Study the drawing (mm; zero at the part's minimum x, y, z) and answer. Coordinates: 2 decimals unless noted, no trailing zeros. Loops run counter-clockwise (first coordinate to the right, second up) from the corner with the lowest first, then second, coordinate; pieces in that order, holes last. Notation, with made-up numbers: (38, 50) - (97, 50) arc R13 ccw to (97, 69) - close; hole circle Ø5 at (-35.75, 67). An arc over 180 degrees is marked (long way). Write each question's results on one line, items separated by ' | '. Start each with the question number.
(1) Find section B-B on x = 59. Determine the outline of the cut face in (y, z).
(2) Given pin 1 Ø2 at (x, z) = (91, 48) entering from -Y; pin 2 Ø1.5 at (x, z) = (64, 31.5) entering from -Y, each flat-ended and moving along its own axis, determine where each tip first touches the part or whether it passes through.
(3) Find section D-D on x = 5. Determine the outline of the cut face in (y, z), then the cut area to 3 significant figures.
(4) Find section C-C on y = 1.8. State how many separate pieces and enclosed holes the cut face has, then the cut area to 3 significant figures.
(5) Consider line 1 (X direction, y = 3.3, z = 48); line 2 (Z direction, x = 81, y = 2.7); line 3 (X direction, y = 1.85, z = 26). Determine where each line is inside the solid, lowest interval first. Write a range as from..to.
(6) Find section A-A on z = 37. Determine the outline of the cut face in (x, y).
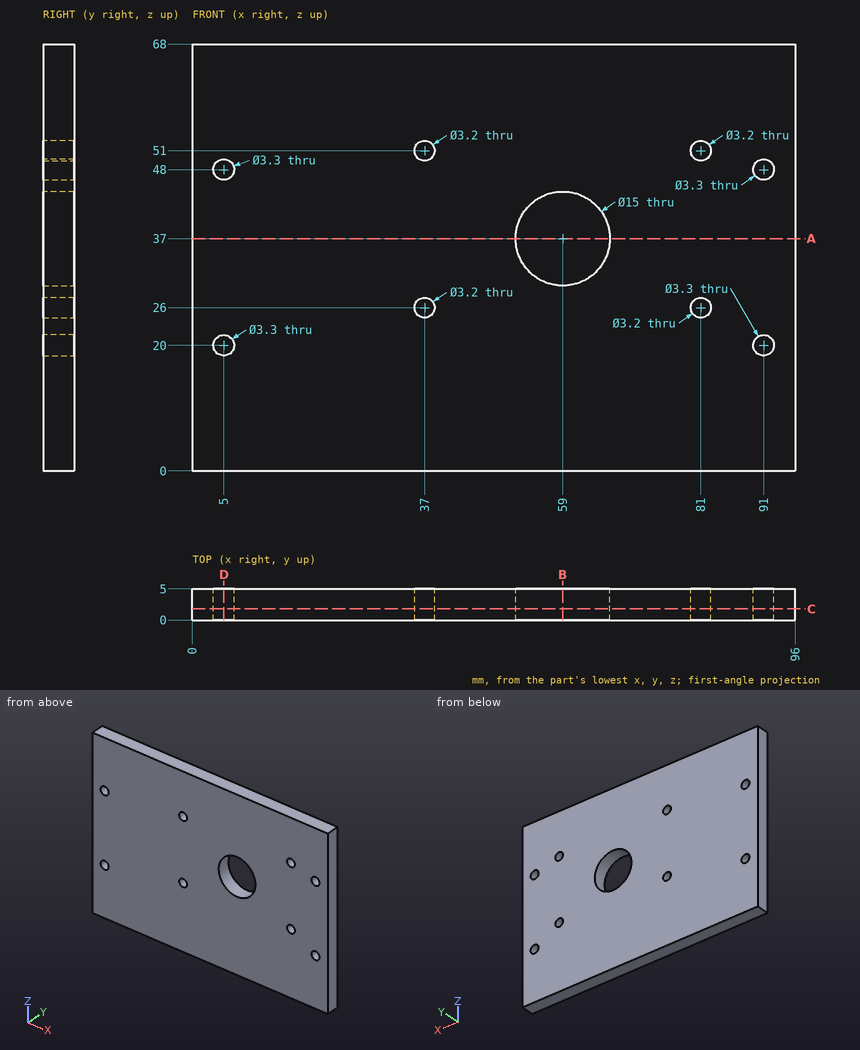
Values:
1) outline: (0, 0) - (5, 0) - (5, 29.5) - (0, 29.5) - close; (0, 44.5) - (5, 44.5) - (5, 68) - (0, 68) - close
2) pin 1: passes through | pin 2: stops at y = 0
3) outline: (0, 0) - (5, 0) - (5, 18.35) - (0, 18.35) - close; (0, 21.65) - (5, 21.65) - (5, 46.35) - (0, 46.35) - close; (0, 49.65) - (5, 49.65) - (5, 68) - (0, 68) - close | area: 307 mm²
4) separate pieces: 1 | enclosed holes: 9 | area: 6,280 mm²
5) line 1: x = 0..3.35, 6.65..89.35, 92.65..96 | line 2: z = 0..24.4, 27.6..49.4, 52.6..68 | line 3: x = 0..35.4, 38.6..79.4, 82.6..96
6) outline: (0, 0) - (51.5, 0) - (51.5, 5) - (0, 5) - close; (66.5, 0) - (96, 0) - (96, 5) - (66.5, 5) - close
